Autodesk Inventor part; units mm, degrees
ref_plane "YZ Plane" through (0, 0, 0) normal (1, 0, 0) x (0, 1, 0)
ref_plane "XZ Plane" through (0, 0, 0) normal (0, 1, 0) x (-1, 0, 0)
ref_plane "XY Plane" through (0, 0, 0) normal (0, 0, 1) x (1, 0, 0)
sketch "Sketch1" plane through (0, 0, 0) normal (0, 0, 1) x (1, 0, 0)
  line L0 (0, 0) -> (50.8, 0)
  line L1 (50.8, 0) -> (50.8, 25.4)
  line L2 (50.8, 25.4) -> (0, 25.4)
  line L3 (0, 25.4) -> (0, 0)
  dimension "d0" = 25.4
  dimension "d1" = 50.8
extrude "Extrusion1" add sketch "Sketch1" along normal blind 635
shell "Shell1" thickness 3.175 removed faces 2 at (16.9333, 16.9333, 0) at (33.8667, 8.4667, 635)
sketch "Sketch2" plane through (0, 25.4, 0) normal (0, 1, 0) x (1, 0, 0)
  line L0 (0, -635) -> (50.8, -635)
  line L1 (50.8, 0) -> (0, 0)
  line L2 (0, 0) -> (0, -635)
  line L3 (12.7, 0) -> (12.7, -50.8) construction
  line L4 (12.7, -50.8) -> (12.7, -101.6) construction
  line L5 (12.7, -101.6) -> (12.7, -533.4) construction
  line L6 (12.7, -533.4) -> (12.7, -584.2) construction
  line L7 (12.7, -584.2) -> (12.7, -635) construction
  circle A0 centre (12.7, -50.8) radius 3.175
  circle A1 centre (12.7, -101.6) radius 3.175
  circle A2 centre (12.7, -533.4) radius 3.175
  circle A3 centre (12.7, -584.2) radius 3.175
  dimension "d4" = 12.7
  dimension "d5" = 50.8
  dimension "d6" = 50.8
  dimension "d7" = 6.35
  dimension "d8" = 6.35
  dimension "d9" = 6.35
  dimension "d10" = 6.35
extrude "Extrusion2" cut sketch "Sketch2" against normal through all
properties part number "Frame_SideRail_Inner_2x1" material "Aluminum-6061"
For this review, take the finished solid that the model builds, in its own axes (mm). A direction names the side the tool comes from. Give positions to 0.01 mm unless a question says otherwise; leave off trailing zeros. Write each loop counter-clockwise with the first axis right and the second up, starting at its lowest first coordinate (ties: lowest second). Pieces come first, ordered by that corner, then holes.
Item 1: The part is to be moulded in two halves that separate along X. For faces 3 (the face through (25, 23, 635)), 4 (the face through (3.175, 13, 313)), 5 (the face through (25, 3.175, 313)), 6 (the face through (0, 13, 313)), say which applies: +X half, -X half, draft (parallel to the pull), parting line (faces both ways), or undercut.
Item 2: Insertion check: P1, Ø5, axis at x = 12.7, z = 533.4, coming from the +Y side. The pin has a flat end and moves straight along its axis. Give the tip position at first contact, or say it passes through.
Item 3: Take a section at C-C (y = 13.25). Give the boundary of the cut face in (x, z) (3 decimals).
Item 4: Take a section at A-A (z = 514). Give the boundary of the cut face in (x, y) (3 decimals).
Item 5: Take a section at B-B (x = 25.5). Give the boundary of the cut face in (y, z) (3 decimals), and give its area (3 significant figures).
Item 6: Wall thickness on probe 1 along Z at (x, y) = (12.7, 23.4) (3 decimals); probe 2 along Y at (x, z) = (20.5, 172) (3 decimals); probe 3 along X at (y, z) = (1.75, 533.4) (3 decimals): over which ranges is each line inside the solid? List them lowest first.
Item 7: Machinability: for faces 1 (the face through (25, 23, 0)), 2 (the face through (26, 22.225, 313)), which of the approach directions +Z, -Z, +X, -X, +Y, -Y give a long, thin tool a straight path to every point of the face, cutting with its end or side? Answer none if there is none.
Established:
1. face 3: draft
1. face 4: undercut
1. face 5: undercut
1. face 6: -X half
2. P1: passes through
3. outline: (0, 0) - (3.175, 0) - (3.175, 635) - (0, 635) - close; (47.625, 0) - (50.8, 0) - (50.8, 635) - (47.625, 635) - close
4. outline: (0, 0) - (50.8, 0) - (50.8, 25.4) - (0, 25.4) - close; hole (3.175, 3.175) - (47.625, 3.175) - (47.625, 22.225) - (3.175, 22.225) - close
5. outline: (0, 0) - (3.175, 0) - (3.175, 635) - (0, 635) - close; (22.225, 0) - (25.4, 0) - (25.4, 635) - (22.225, 635) - close
5. area: 4,030 mm2
6. probe 1: z = 0 to 47.625, 53.975 to 98.425, 104.775 to 530.225, 536.575 to 581.025, 587.375 to 635
6. probe 2: y = 0 to 3.175, 22.225 to 25.4
6. probe 3: x = 0 to 9.525, 15.875 to 50.8
7. face 1: -Z, +X, -X, +Y, -Y
7. face 2: +Z, -Z
